from build123d import *

# Parameters (mm, degrees)
BOSS_EXTRUDE1_DEPTH = 960
SKETCH2_R           = 12.7
BOSS_EXTRUDE2_DEPTH = 5


with BuildPart() as part:
    # Sketch1 → Boss-Extrude1 (new body)
    with BuildSketch(Plane.XY):
        with BuildLine():
            Line((-324.9668, 16.7), (324.9668, 16.7))
            ThreePointArc((324.9668, 16.7), (341.6668, 0), (324.9668, -16.7))
            Line((324.9668, -16.7), (-324.9668, -16.7))
            ThreePointArc((-324.9668, -16.7), (-341.6668, 0), (-324.9668, 16.7))
        make_face()
        with BuildLine():
            Line((-324.9668, 12.7), (324.9668, 12.7))
            ThreePointArc((324.9668, 12.7), (337.6668, 0), (324.9668, -12.7))
            Line((324.9668, -12.7), (-324.9668, -12.7))
            ThreePointArc((-324.9668, -12.7), (-337.6668, 0), (-324.9668, 12.7))
        make_face(mode=Mode.SUBTRACT)
    extrude(amount=BOSS_EXTRUDE1_DEPTH)

    # Sketch2 → Boss-Extrude2 (add)
    with BuildSketch(Plane.XY.offset(960)):
        with BuildLine():
            Line((-324.9668, 30), (324.9668, 30))
            ThreePointArc((324.9668, 30), (354.9668, 0), (324.9668, -30))
            Line((324.9668, -30), (-324.9668, -30))
            ThreePointArc((-324.9668, -30), (-354.9668, 0), (-324.9668, 30))
        make_face()
        with Locations(Location((324.9668, 0, 0), (0, 0, 90))):
            Circle(SKETCH2_R, mode=Mode.SUBTRACT)
        with Locations(Location((-324.9668, 0, 0), (0, 0, 270))):
            Circle(SKETCH2_R, mode=Mode.SUBTRACT)
    boss_extrude2 = extrude(amount=BOSS_EXTRUDE2_DEPTH)

    # Mirror1: Boss-Extrude2 across plane
    add(boss_extrude2.mirror(Plane.XY.offset(480)))


solid = part.part
Read the model definition and answer for the solid it produces. Units are mm, in the model's axes. A direction names the side the tool comes from. Give positions to 0.01 mm unless a question says otherwise; leave off trailing zeros. Write each loop counter-clockwise with the first axis right and the second up, starting at its lowest first coordinate (ties: lowest second). Pieces come first, ordered by that corner, then holes. Notation, with made-up numbers: (9.25, -31.5) - (48.25, -31.5) arc R34 ccw to (48.25, 0.5) - close; hole circle Ø1 at (49, 68). An arc over 180 degrees is marked (long way). Answer in a Markdown table with one row per item. Add a question column.
Item 1: Section A-A, the plane x = -192 is taken. Write down the section's boundary in (y, z).
Item 2: Section B-B, the plane z = 623 is taken. Write down the section's boundary in (x, y).
Item 3: Section C-C, the plane y = 0 is taken. Write down the section's boundary in (x, z), and give its area (3 significant figures).
Item 4: Find the intervals of material crossed by L1, parallel to Z at x = -194.5, y = -27; L2, parallel to X at y = 0, z = 512; L3, parallel to Y at x = 100, z = 591, in increasing order.
Item 5: A tool of negligible diameter and unlimited length cuts with its end or side. For faces 4 (the face through (5, -16.7, 473)), 5 (the face through (-341.663, -0.367, 473.28)), 6 (the face through (337.365, -2.753, 486.79)), 7 (the face through (5, 0, 960)), from which of +Z, -Z, +X, -X, +Y, -Y can it reach the whole face along a straight path? Write none if from no direction.
Item 6: Flat-ended cylindrical pins translate along their axes: P1, Ø3, axis at x = -93.5, z = 512, coming from the +Y side; P2, Ø5, axis at x = -168, z = 209.5, coming from the -Y side. Find the tip coordinate at first contact, or state that the pin passes through.
Item 7: Determine the mould class of faces 1 (the face through (341.663, 0.367, 473.28)), 2 (the face through (-337.365, 2.753, 486.79)), 3 (the face through (-354.96, -0.66, 962.46)) for opening direction X: pulls with the +X half, pulls with the -X half, needs draft (parallel to the pull), parting line crosses it, or undercut.
Recorded:
| question | item | result |
|---|---|---|
| 1 | outline | (-30, -5) - (30, -5) - (30, 0) - (16.7, 0) - (16.7, 960) - (30, 960) - (30, 965) - (-30, 965) - (-30, 960) - (-16.7, 960) - (-16.7, 0) - (-30, 0) - close; hole (-12.7, 0) - (12.7, 0) - (12.7, 960) - (-12.7, 960) - close |
| 2 | outline | (-324.97, -16.7) - (324.97, -16.7) arc R16.7 ccw to (324.97, 16.7) - (-324.97, 16.7) arc R16.7 ccw to start; hole (-324.97, -12.7) - (324.97, -12.7) arc R12.7 ccw to (324.97, 12.7) - (-324.97, 12.7) arc R12.7 ccw to start |
| 3 | outline | (-354.97, -5) - (-337.67, -5) - (-337.67, 965) - (-354.97, 965) - (-354.97, 960) - (-341.67, 960) - (-341.67, 0) - (-354.97, 0) - close; (-312.27, -5) - (312.27, -5) - (312.27, 0) - (-312.27, 0) - close; (-312.27, 960) - (312.27, 960) - (312.27, 965) - (-312.27, 965) - close; (337.67, -5) - (354.97, -5) - (354.97, 0) - (341.67, 0) - (341.67, 960) - (354.97, 960) - (354.97, 965) - (337.67, 965) - close |
| 3 | area | 14,300 mm2 |
| 4 | L1 | z = -5 to 0, 960 to 965 |
| 4 | L2 | x = -341.67 to -337.67, 337.67 to 341.67 |
| 4 | L3 | y = -16.7 to -12.7, 12.7 to 16.7 |
| 5 | face 4 | +X, -X, -Y |
| 5 | face 5 | -X |
| 5 | face 6 | +Z, -Z |
| 5 | face 7 | none |
| 6 | P1 | stops at y = 16.7 |
| 6 | P2 | stops at y = -16.7 |
| 7 | face 1 | pulls with the +X half |
| 7 | face 2 | undercut |
| 7 | face 3 | pulls with the -X half |
